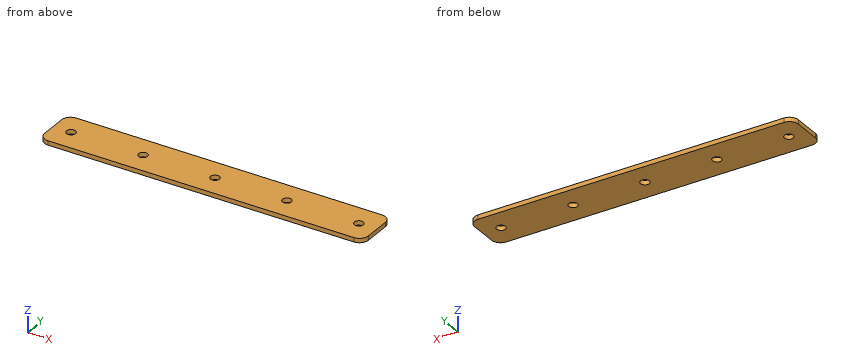
Autodesk Inventor part; units mm, degrees
ref_plane "YZ Plane" through (0, 0, 0) normal (1, 0, 0) x (0, 1, 0)
ref_plane "XZ Plane" through (0, 0, 0) normal (0, 1, 0) x (-1, 0, 0)
ref_plane "XY Plane" through (0, 0, 0) normal (0, 0, 1) x (1, 0, 0)
sketch "Sketch1" plane through (0, 0, 0) normal (0, 0, 1) x (1, 0, 0)
  line L0 (0, 0) -> (228.6, 0)
  line L1 (228.6, 0) -> (228.6, 31.75)
  line L2 (228.6, 31.75) -> (0, 31.75)
  line L3 (0, 31.75) -> (0, 0)
  circle A0 centre (215.9, 15.875) radius 3.1623
  line L4 (-50.8, 0) -> (177.8, 0)
  circle A1 centre (165.1, 15.875) radius 3.1623
  line L5 (-101.6, 0) -> (127, 0)
  circle A2 centre (114.3, 15.875) radius 3.1623
  line L6 (-152.4, 0) -> (76.2, 0)
  circle A3 centre (63.5, 15.875) radius 3.1623
  line L7 (-203.2, 0) -> (25.4, 0)
  circle A4 centre (12.7, 15.875) radius 3.1623
  dimension "d0" = 228.6
  dimension "d1" = 31.75
  dimension "d2" = 6.3246
  dimension "d3" = 12.7
  dimension "d4" = 15.875
  dimension "d7" = 50.8
extrude "Plate1" add sketch "Sketch1" along normal blind 3.048
fillet "Corner Round1" radius 6.35 4 edges at (228.6, 31.75, 1.524) (228.6, 0, 1.524) (0, 31.75, 1.524) (0, 0, 1.524)
equation "\"BendRadius\" = Thickness"
equation "\"BendReliefWidth\" = Thickness"
equation "\"BendReliefDepth\" = 0.5 * Thickness"
equation "\"CornerReliefSize\" = 4 * Thickness"
equation "\"MinimumRemnant\" = 2 * Thickness"
equation "\"TransitionRadius\" = BendRadius"
equation "\"JacobiRadiusSize\" = BendRadius"
equation "\"GapSize\" = Thickness"
equation "\"d12\" = BendRadius"
properties part number "super3"
Can you work these out from the model? Positions are in its coordinate system, mm. Coordinates: 2 decimals unless noted, no trailing zeros. Write each loop counter-clockwise with the first axis right and the second up, starting at its lowest first coordinate (ties: lowest second). Pieces come first, ordered by that corner, then holes.
Q1. Imagine slicing it at A-A, the plane x = 215.9. List the corners of the cut face in (y, z) for me, plus the area to 3 significant figures.
Results found:
outline: (0, 0) - (12.71, 0) - (12.71, 3.05) - (0, 3.05) - close; (19.04, 0) - (31.75, 0) - (31.75, 3.05) - (19.04, 3.05) - close
area: 77.5 mm2
Q2. Please list where these lines run through material, in increasing order: L1, parallel to X at y = 13, z = 0.35; L2, parallel to X at y = 13.5, z = 1.7; L3, parallel to Y at x = 215.9, z = 1.35.
Results found:
L1: x = 0 to 11.38, 14.02 to 62.18, 64.82 to 112.98, 115.62 to 163.78, 166.42 to 214.58, 217.22 to 228.6
L2: x = 0 to 10.61, 14.79 to 61.41, 65.59 to 112.21, 116.39 to 163.01, 167.19 to 213.81, 217.99 to 228.6
L3: y = 0 to 12.71, 19.04 to 31.75
Q3. For P1, Ø5, axis at x = 63.5, y = 15.875, coming from the -Z side; P2, Ø1.5, axis at y = 6, z = 2.5, coming from the -X side, each with a flat end and sliding along its axis, tell me the tip position at first contact or that it passes through.
Results found:
P1: passes through
P2: stops at x = 0
Q4. Imagine slicing it at B-B, the plane z = 1.4. List the corners of the cut face in (x, y) for me (3 decimals).
Results found:
outline: (0, 6.35) arc R6.35 ccw to (6.35, 0) - (222.25, 0) arc R6.35 ccw to (228.6, 6.35) - (228.6, 25.4) arc R6.35 ccw to (222.25, 31.75) - (6.35, 31.75) arc R6.35 ccw to (0, 25.4) - close; hole circle Ø6.325 at (12.7, 15.875); hole circle Ø6.325 at (63.5, 15.875); hole circle Ø6.325 at (114.3, 15.875); hole circle Ø6.325 at (165.1, 15.875); hole circle Ø6.325 at (215.9, 15.875)
